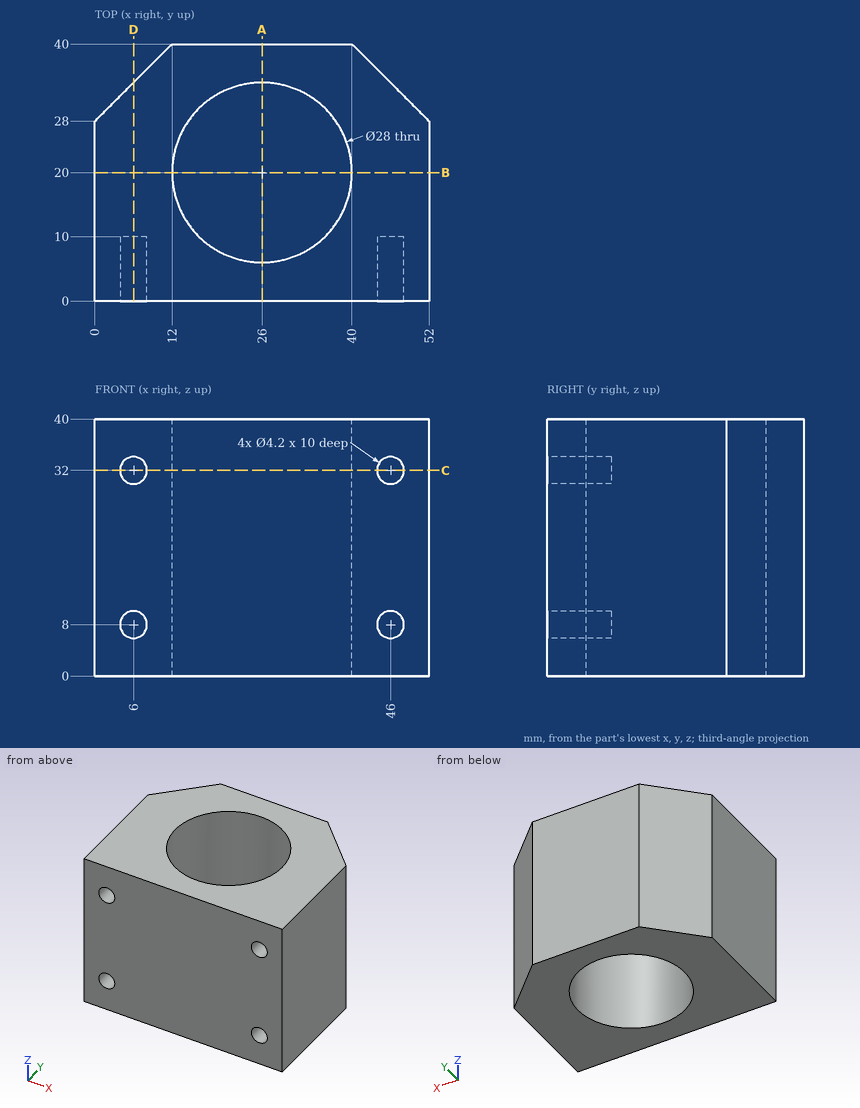
Design review of the part shown in the three views and the two pictorial views. Dimensions are in mm from the part's minimum x, y and z. Give positions to 0.01 mm unless a question says otherwise; leave off trailing zeros. Loops run counter-clockwise (first coordinate to the right, second up) from the corner with the lowest first, then second, coordinate; pieces in that order, holes last. Notation, with made-up numbers: M 84.25,8 L 88.25,8 A23 cw 88.25,27 Z; hole C -27.5,75.5 d10. An arc over 180 degrees is marked long. Put each result on its own line as item: value. Start each with the question number.
(1) For pin 1 (2 mm diameter, centred on x = 46, z = 7, fed in from -Y); pin 2 (6.5 mm diameter, centred on x = 6, z = 32, fed in from +Y), all flat-tipped, find the tip position at first contact; note any pin that passes through.
(2) Add section D-D, the plane x = 6. Write out the cut boundary in (y, z).
(3) Add section C-C, the plane z = 32. Write out the cut boundary in (x, y), then the cut area to 3 significant figures.
(4) Add section A-A, the plane x = 26. Write out the cut boundary in (y, z).
(5) Add section B-B, the plane y = 20. Write out the cut boundary in (x, z).
(6) Wall thickness on L1, parallel to Z at x = 46, y = 6.75; L2, parallel to Y at x = 26, z = 15; L3, parallel to X at y = 32.5, z = 32: over which ranges is each line inside the solid? List them lowest first.
Result:
1. pin 1: stops at y = 10
1. pin 2: stops at y = 37.25
2. outline: M 0,0 L 34,0 L 34,40 L 0,40 L 0,34.1 L 10,34.1 L 10,29.9 L 0,29.9 L 0,10.1 L 10,10.1 L 10,5.9 L 0,5.9 Z
3. outline: M 0,0 L 3.9,0 L 3.9,10 L 8.1,10 L 8.1,0 L 43.9,0 L 43.9,10 L 48.1,10 L 48.1,0 L 52,0 L 52,28 L 40,40 L 12,40 L 0,28 Z; hole C 26,20 d28
3. area: 1,240 mm^2
4. outline: M 0,0 L 6,0 L 6,40 L 0,40 Z; M 34,0 L 40,0 L 40,40 L 34,40 Z
5. outline: M 0,0 L 12,0 L 12,40 L 0,40 Z; M 40,0 L 52,0 L 52,40 L 40,40 Z
6. L1: z = 0 to 5.9, 10.1 to 29.9, 34.1 to 40
6. L2: y = 0 to 6, 34 to 40
6. L3: x = 4.5 to 19.7, 32.3 to 47.5
